Read the model definition and answer for the solid it produces. Units are mm, in the model's axes. A direction names the side the tool comes from. Round coordinates to 2 decimals unless told otherwise and drop trailing zeros. Write each loop counter-clockwise with the first axis right and the second up, starting at its lowest first coordinate (ties: lowest second). Pieces come first, ordered by that corner, then holes. Notation, with made-up numbers: (-21.5, -15.5) - (-9.5, -15.5) arc R30 ccw to (-9.5, 15.5) - close; hole circle Ø3 at (40.5, 22.25). An arc over 180 degrees is marked (long way). One line per item, written item: value. Start each with the question number.
(1) Find the intervals of material crossed by L1, parallel to X at y = 39, z = 94; L2, parallel to Y at x = 10, z = 168.5; L3, parallel to Y at x = 15.5, z = 60, in increasing order.
(2) A cutting plane is placed at D-D, the plane y = 36.5. Determine the outline of the cut face in (x, z).
(3) A cutting plane is placed at B-B, the plane z = 168.5. Determine the outline of the cut face in (x, y), plus the area to 3 significant figures.
(4) The mould has two halves that part along Y. Classify faces 3 (the face through (4.674, 38, 122)), 4 (the face through (20, 76.2, 122)), 5 (the face through (20, 0, 122)), 6 (the face through (4, 38, 0)): +Y half, -Y half, draft (parallel to the pull), parting line (faces both ways), or undercut.
(5) A cutting plane is placed at C-C, the plane x = 33. Determine the outline of the cut face in (y, z).
(6) Flat-ended cylindrical pins translate along their axes: pin 1 Ø6 at (y, z) = (43, 63) entering from -X; pin 2 Ø13 at (y, z) = (43, 92) entering from +X. Find the tip coordinate at first contact, or state that the pin passes through.
(7) A cutting plane is placed at A-A, the plane x = 23. Determine the outline of the cut face in (y, z), plus the area to 3 significant figures.
(8) For faces 1 (the face through (24.07, 7.25, 122.09)), 2 (the face through (0, 38, 122)), determine the directions among +Z, -Z, +X, -X, +Y, -Y from which every point of the face is accessible in a straight line to the end or side of a thin tool.
from build123d import *

# Parameters (mm, degrees)
BOSS_EXTRUDE1_DEPTH = 247.65


with BuildPart() as part:
    # Sketch1 → Boss-Extrude1 (new body)
    with BuildSketch(Plane.XY):
        with BuildLine():
            Line((0, 0), (0, 76.2))
            Line((0, 76.2), (40.2336, 76.2))
            Line((40.2336, 76.2), (40.2336, 74.011994208))
            ThreePointArc((40.2336, 74.011994208), (39.571488513, 72.206035358), (37.898963373, 71.256015019))
            Line((37.898963373, 71.256015019), (10.616311414, 66.708574647))
            ThreePointArc((10.616311414, 66.708574647), (6.358974694, 64.290341057), (4.6736, 59.693354893))
            Line((4.6736, 59.693354893), (4.6736, 16.506645107))
            ThreePointArc((4.6736, 16.506645107), (6.358974694, 11.909658943), (10.616311414, 9.491425353))
            Line((10.616311414, 9.491425353), (37.898963373, 4.943984981))
            ThreePointArc((37.898963373, 4.943984981), (39.571488513, 3.993964642), (40.2336, 2.188005792))
            Line((40.2336, 2.188005792), (40.2336, 0))
            Line((40.2336, 0), (0, 0))
        make_face()
    extrude(amount=BOSS_EXTRUDE1_DEPTH)


solid = part.part
Here are the results:
1. L1: 0 to 4.67
1. L2: 0 to 9.62, 66.58 to 76.2
1. L3: 0 to 8.68, 67.52 to 76.2
2. outline: (0, 0) - (4.67, 0) - (4.67, 247.65) - (0, 247.65) - close
3. outline: (0, 0) - (40.23, 0) - (40.23, 2.19) arc R2.79 ccw to (37.9, 4.94) - (10.62, 9.49) arc R7.11 cw to (4.67, 16.51) - (4.67, 59.69) arc R7.11 cw to (10.62, 66.71) - (37.9, 71.26) arc R2.79 ccw to (40.23, 74.01) - (40.23, 76.2) - (0, 76.2) - close
3. area: 903 mm²
4. face 3: undercut
4. face 4: +Y half
4. face 5: -Y half
4. face 6: draft
5. outline: (0, 0) - (5.76, 0) - (5.76, 247.65) - (0, 247.65) - close; (70.44, 0) - (76.2, 0) - (76.2, 247.65) - (70.44, 247.65) - close
6. pin 1: x = 0
6. pin 2: x = 4.67
7. outline: (0, 0) - (7.43, 0) - (7.43, 247.65) - (0, 247.65) - close; (68.77, 0) - (76.2, 0) - (76.2, 247.65) - (68.77, 247.65) - close
7. area: 3,680 mm²
8. face 1: +Z, -Z, +X
8. face 2: +Z, -Z, -X, +Y, -Y
